Geometry check sheet. Reference: the model listing, model coordinates, mm. A direction names the side the tool comes from. Round coordinates to 2 decimals unless told otherwise and drop trailing zeros. Order: outer loops, then holes, each group sorted by start corner. A loop starts at its lowest first (then second) coordinate and runs counter-clockwise, first axis right, second up.
(1) Go/stop test with flat-tipped pins: pin 1 (4 mm diameter, centred on x = 6.5, z = 0, fed in from +Y); pin 2 (1 mm diameter, centred on x = 7.5, y = 6, fed in from -Z). Record where each tip stops, or that it passes through.
(2) Sectioned sample at B-B (x = -3.75). Record the boundary of the cut face in (y, z).
(3) Set-up check for faces 4 (the face through (-6.854, 4.535, -0.01)), 5 (the face through (-7.7, 4.5, -4.9)): record each of +Z, -Z, +X, -X, +Y, -Y from which the full face is reachable in a straight line by a thin tool's end or side.
(4) Sectioned sample at A-A (z = 5.5). Record the boundary of the cut face in (x, y).
(5) Material ranges on line 1 along Z through (x, y) = (-5.5, 4.65); line 2 along X through (y, z) = (5.3, -5.5); line 3 along X through (y, z) = (4.5, -1.5), recorded low to high.
(6) Release check for a two-part mould opening along X. For faces 1 (the face through (-9.356, 4.465, -1.561)), 2 (the face through (4.302, 4.535, -4.431)), 3 (the face through (2.561, 4.465, -8.356)) record: +X half, -X half, draft (parallel to the pull), parting line (faces both ways), or undercut.
from build123d import *

# Parameters (mm, degrees)
SKETCH1_W             = 20
SKETCH1_H             = 20
SKETCH1_R             = 4
SKETCH1_H_2           = 10
BOSS_EXTRUDE2_DEPTH   = 2
SKETCH2_W             = 45
SKETCH2_H             = 60
SKETCH2_W_2           = 43
SKETCH2_H_2           = 58
BOSS_EXTRUDE3_DEPTH   = 4
SKETCH6_W             = 45
SKETCH6_H             = 30
BOSS_EXTRUDE4_DEPTH   = 2
CUT_EXTRUDE4_DEPTH    = 4
BOSS_EXTRUDE5_DEPTH   = 7
BOSS_EXTRUDE5_2_DEPTH = 7
BOSS_EXTRUDE5_3_DEPTH = 7
SKETCH14_R            = 4
CUT_EXTRUDE7_DEPTH    = 19
SKETCH20_R            = 9.7
BOSS_EXTRUDE6_DEPTH   = 5
CUT_EXTRUDE8_DEPTH    = 15
CUT_EXTRUDE9_DEPTH    = 15
CUT_EXTRUDE10_DEPTH   = 31
SKETCH24_W            = 45
SKETCH24_H            = 30
CUT_EXTRUDE11_DEPTH   = 31
SKETCH25_W            = 45
SKETCH25_H            = 60
CUT_EXTRUDE12_DEPTH   = 31
SKETCH26_R            = 1
CUT_EXTRUDE14_DEPTH   = 31
SKETCH28_R            = 8.330942509
BOSS_EXTRUDE7_DEPTH   = 5
CUT_EXTRUDE15_DEPTH   = 10


with BuildPart() as part:
    # Sketch1 → Boss-Extrude2 (new body)
    # profile 1 of 6: a face of its own
    with BuildSketch(Plane(origin=(0, 0, 0), x_dir=(1, 0, 0), z_dir=(0, 1, 0))):
        Polygon((-22.5, 10), (-10, 10), (10, 10), (22.5, 10), (22.5, 70), (-22.5, 70), align=None)
    # profile 2 of 6: a face of its own
    with BuildSketch(Plane(origin=(0, 0, 0), x_dir=(1, 0, 0), z_dir=(0, 1, 0))):
        Polygon((-22.5, 10), (-10, -10), (-10, 10), align=None)
    # profile 3 of 6: a face of its own
    with BuildSketch(Plane(origin=(0, 0, 0), x_dir=(1, 0, 0), z_dir=(0, 1, 0))):
        Polygon((10, 10), (10, -10), (22.5, 10), align=None)
    # profile 4 of 6: a face of its own
    with BuildSketch(Plane(origin=(0, 0, 0), x_dir=(1, 0, 0), z_dir=(0, 1, 0))):
        Rectangle(SKETCH1_W, SKETCH1_H)
        Circle(SKETCH1_R, mode=Mode.SUBTRACT)
    # profile 5 of 6: a face of its own
    with BuildSketch(Plane(origin=(0, 0, 0), x_dir=(1, 0, 0), z_dir=(0, 1, 0))):
        Circle(SKETCH1_R)
    # profile 6 of 6: a face of its own
    with BuildSketch(Plane(origin=(0, 0, 0), x_dir=(1, 0, 0), z_dir=(0, 1, 0))):
        with Locations((0, -15)):
            Rectangle(SKETCH1_W, SKETCH1_H_2)
    extrude(amount=BOSS_EXTRUDE2_DEPTH)

    # Sketch2 → Boss-Extrude3 (add)
    with BuildSketch(Plane(origin=(0, 2, 0), x_dir=(1, 0, 0), z_dir=(0, 1, 0))):
        with Locations((0, 40)):
            Rectangle(SKETCH2_W, SKETCH2_H)
        with Locations((0, 40)):
            Rectangle(SKETCH2_W_2, SKETCH2_H_2, mode=Mode.SUBTRACT)
    extrude(amount=BOSS_EXTRUDE3_DEPTH)

    # Sketch6 → Boss-Extrude4 (add)
    with BuildSketch(Plane(origin=(0, 2, 0), x_dir=(1, 0, 0), z_dir=(0, 1, 0))):
        with Locations((0, -5)):
            Rectangle(SKETCH6_W, SKETCH6_H)
    extrude(amount=-BOSS_EXTRUDE4_DEPTH)

    # Sketch7 → Cut-Extrude4 (cut)
    with BuildSketch(Plane(origin=(0, 2, 0), x_dir=(1, 0, 0), z_dir=(0, 1, 0))):
        with BuildLine():
            Line((9.5, 9.5), (-9.5, 9.5))
            Line((-9.5, 9.5), (-9.5, 2.122498999))
            ThreePointArc((-9.5, 2.122498999), (0, 9), (9.5, 2.122498999))
            Line((9.5, 2.122498999), (9.5, 9.5))
        make_face()
        with BuildLine():
            ThreePointArc((-5.267826876, -9.5), (-7.858215886, -7.184532568), (-9.5, -4.122498999))
            Line((-9.5, -4.122498999), (-9.5, -9.5))
            Line((-9.5, -9.5), (-5.267826876, -9.5))
        make_face()
        with BuildLine():
            Line((9.5, -9.5), (9.5, -4.122498999))
            ThreePointArc((9.5, -4.122498999), (7.858215886, -7.184532568), (5.267826876, -9.5))
            Line((5.267826876, -9.5), (9.5, -9.5))
        make_face()
    extrude(amount=-CUT_EXTRUDE4_DEPTH, mode=Mode.SUBTRACT)

    # Sketch14 → Cut-Extrude7 (cut)
    with BuildSketch(Plane.XZ):
        with Locations(Location((0, 1, 0), (0, 0, 270))):
            Circle(SKETCH14_R)
    extrude(amount=-CUT_EXTRUDE7_DEPTH, mode=Mode.SUBTRACT)

    # Sketch20 → Boss-Extrude6 (add)
    with BuildSketch(Plane(origin=(0, 2, 0), x_dir=(1, 0, 0), z_dir=(0, 1, 0))):
        with Locations(Location((0, -1, 0), (0, 0, 270))):
            Circle(SKETCH20_R)
        Polygon((7.160405698, -4.567714988), (7.585926887, 1.540415964), (3.567714988, 6.160405698), (-2.540415964, 6.585926887), (-7.160405698, 2.567714988), (-7.585926887, -3.540415964), (-3.567714988, -8.160405698), (2.540415964, -8.585926887), align=None, mode=Mode.SUBTRACT)
    extrude(amount=BOSS_EXTRUDE6_DEPTH)

    # Sketch24 → Cut-Extrude11 (cut)
    with BuildSketch(Plane(origin=(0, 2, 0), x_dir=(1, 0, 0), z_dir=(0, 1, 0))):
        with Locations((0, -5)):
            Rectangle(SKETCH24_W, SKETCH24_H)
    extrude(amount=-CUT_EXTRUDE11_DEPTH, mode=Mode.SUBTRACT)


with BuildPart() as body_2:
    # Sketch8 → Boss-Extrude5 (new body)
    with BuildSketch(Plane(origin=(0, 2, 0), x_dir=(1, 0, 0), z_dir=(0, 1, 0))):
        with BuildLine():
            Line((9.5, 2.122498999), (9.5, 9.5))
            Line((9.5, 9.5), (-9.5, 9.5))
            Line((-9.5, 9.5), (-9.5, 2.122498999))
            ThreePointArc((-9.5, 2.122498999), (0, 9), (9.5, 2.122498999))
        make_face()
    extrude(amount=BOSS_EXTRUDE5_DEPTH)

    # Sketch21 → Cut-Extrude8 (cut)
    with BuildSketch(Plane(origin=(0, 9, 0), x_dir=(1, 0, 0), z_dir=(0, 1, 0))):
        with BuildLine():
            Line((-9.5, 9.5), (-9.5, 2.122498999))
            ThreePointArc((-9.5, 2.122498999), (0, 9), (9.5, 2.122498999))
            Line((9.5, 2.122498999), (9.5, 9.5))
            Line((9.5, 9.5), (-9.5, 9.5))
        make_face()
    extrude(amount=-CUT_EXTRUDE8_DEPTH, mode=Mode.SUBTRACT)


with BuildPart() as body_3:
    # Sketch8 → Boss-Extrude5 2 (new body)
    with BuildSketch(Plane(origin=(0, 2, 0), x_dir=(1, 0, 0), z_dir=(0, 1, 0))):
        with BuildLine():
            Line((-9.5, -9.5), (-5.267826876, -9.5))
            ThreePointArc((-5.267826876, -9.5), (-7.858215886, -7.184532568), (-9.5, -4.122498999))
            Line((-9.5, -4.122498999), (-9.5, -9.5))
        make_face()
    extrude(amount=BOSS_EXTRUDE5_2_DEPTH)

    # Sketch22 → Cut-Extrude9 (cut)
    with BuildSketch(Plane(origin=(0, 9, 0), x_dir=(1, 0, 0), z_dir=(0, 1, 0))):
        with BuildLine():
            Line((-9.5, -4.122498999), (-9.5, -9.5))
            Line((-9.5, -9.5), (-5.267826876, -9.5))
            ThreePointArc((-5.267826876, -9.5), (-7.858215886, -7.184532568), (-9.5, -4.122498999))
        make_face()
    extrude(amount=-CUT_EXTRUDE9_DEPTH, mode=Mode.SUBTRACT)


with BuildPart() as body_4:
    # Sketch8 → Boss-Extrude5 3 (new body)
    with BuildSketch(Plane(origin=(0, 2, 0), x_dir=(1, 0, 0), z_dir=(0, 1, 0))):
        with BuildLine():
            Line((9.5, -9.5), (9.5, -4.122498999))
            ThreePointArc((9.5, -4.122498999), (7.858215886, -7.184532568), (5.267826876, -9.5))
            Line((5.267826876, -9.5), (9.5, -9.5))
        make_face()
    extrude(amount=BOSS_EXTRUDE5_3_DEPTH)

    # Sketch23 → Cut-Extrude10 (cut)
    with BuildSketch(Plane(origin=(0, 9, 0), x_dir=(1, 0, 0), z_dir=(0, 1, 0))):
        with BuildLine():
            Line((5.267826876, -9.5), (9.5, -9.5))
            Line((9.5, -9.5), (9.5, -4.122498999))
            ThreePointArc((9.5, -4.122498999), (7.858215886, -7.184532568), (5.267826876, -9.5))
        make_face()
    extrude(amount=-CUT_EXTRUDE10_DEPTH, mode=Mode.SUBTRACT)


with BuildPart() as cut_extrude11_piece_1:
    # of the separate pieces the step leaves, piece 1, a body of its own (cut_extrude11_pieces)
    add(part.part.solids().sort_by_distance((-22.5, 0, -10))[0])

    # Sketch25 → Cut-Extrude12 (cut)
    with BuildSketch(Plane(origin=(0, 6, 0), x_dir=(1, 0, 0), z_dir=(0, 1, 0))):
        with Locations((0, 40)):
            Rectangle(SKETCH25_W, SKETCH25_H)
    extrude(amount=-CUT_EXTRUDE12_DEPTH, mode=Mode.SUBTRACT)


with BuildPart() as cut_extrude11_piece_2:
    # of the separate pieces the step leaves, piece 2, a body of its own (cut_extrude11_pieces)
    add(part.part.solids().sort_by_distance((0, 2, 10.7))[0])

    # Sketch26 → Cut-Extrude14 (cut)
    with BuildSketch(Plane(origin=(0, 7, 0), x_dir=(1, 0, 0), z_dir=(0, 1, 0))):
        with Locations((0.674113898, 8.676547445)):
            Circle(SKETCH26_R)
        with Locations((-6.365681808, 6.319022826)):
            Circle(SKETCH26_R)
        with Locations((-9.676547445, -0.325886102)):
            Circle(SKETCH26_R)
        with Locations((-8.681991909, 3.325854423)):
            Circle(SKETCH26_R)
        with Locations((-9.19793635, -4.080254356)):
            Circle(SKETCH26_R)
        with Locations((-7.319022826, -7.365681808)):
            Circle(SKETCH26_R)
        with Locations((-4.325854423, -9.681991909)):
            Circle(SKETCH26_R)
        with Locations((-0.674113898, -10.676547445)):
            Circle(SKETCH26_R)
        with Locations((3.080254356, -10.19793635)):
            Circle(SKETCH26_R)
        with Locations((6.365681808, -8.319022826)):
            Circle(SKETCH26_R)
        with Locations((8.681991909, -5.325854423)):
            Circle(SKETCH26_R)
        with Locations((9.676547445, -1.674113898)):
            Circle(SKETCH26_R)
        with Locations((9.19793635, 2.080254356)):
            Circle(SKETCH26_R)
        with Locations((7.319022826, 5.365681808)):
            Circle(SKETCH26_R)
        with Locations((4.325854423, 7.681991909)):
            Circle(SKETCH26_R)
        with Locations((-3.080254356, 8.19793635)):
            Circle(SKETCH26_R)
    extrude(amount=-CUT_EXTRUDE14_DEPTH, mode=Mode.SUBTRACT)

    # Sketch28 → Boss-Extrude7 (add)
    with BuildSketch(Plane(origin=(0, 7, 0), x_dir=(1, 0, 0), z_dir=(0, 1, 0))):
        with Locations((0, -1)):
            Circle(SKETCH28_R)
    extrude(amount=-BOSS_EXTRUDE7_DEPTH)

    # Sketch29 → Cut-Extrude15 (cut)
    with BuildSketch(Plane(origin=(0, 7, 0), x_dir=(1, 0, 0), z_dir=(0, 1, 0))):
        Polygon((-6.311211771, 3.916157644), (-7.413123294, -4.0075909), (-1.101911524, -8.923748544), (6.311211771, -5.916157644), (7.413123294, 2.0075909), (1.101911524, 6.923748544), align=None)
    extrude(amount=-CUT_EXTRUDE15_DEPTH, mode=Mode.SUBTRACT)


solid = cut_extrude11_piece_2.part
Answer below:
1. pin 1: stops at y = 7
1. pin 2: stops at z = -4.58
2. outline: (2, -7.46) - (7, -7.46) - (7, -4.96) - (2, -4.96) - close; (2, 6.86) - (7, 6.86) - (7, 8.86) - (2, 8.86) - close
3. face 4: +Y, -Y
3. face 5: -Z, -X, +Y, -Y
4. outline: (-8.59, 2) - (-5.5, 2) - (-5.5, 7) - (-8.59, 7) - close; (6.37, 2) - (7.7, 2) - (7.7, 7) - (6.37, 7) - close
5. line 1: z = -6.99 to -6.82, -5.82 to -4.25, 5.5 to 8.99
5. line 2: x = -7.2 to -6.94, -5.79 to -2.41, 2.93 to 6.33
5. line 3: x = -9.37 to -6.65, 7.34 to 8.38
6. face 1: -X half
6. face 2: undercut
6. face 3: +X half
